Could you check a few things on this drawing? It's one solid part, dimensions in mm from its lowest x, y, z. A direction names the side the tool comes from. Give positions to 0.01 mm unless a question says otherwise; leave off trailing zeros. Order: outer loops, then holes, each group sorted by start corner. A loop starts at its lowest first (then second) coordinate and runs counter-clockwise, first axis right, second up.
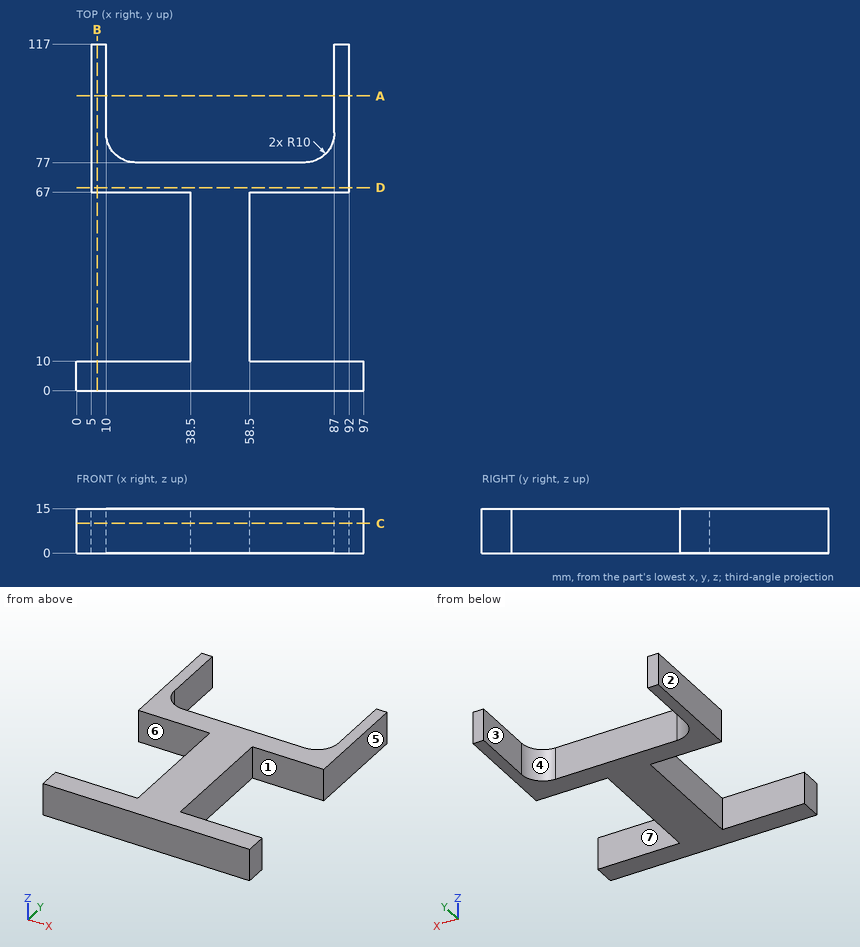
Item 1: Imagine slicing it at A-A on y = 99.5. List the corners of the cut face in (x, z) for me.
Findings:
outline: (5, 0) - (10, 0) - (10, 15) - (5, 15) - close; (87, 0) - (92, 0) - (92, 15) - (87, 15) - close
Item 2: For the marked faces 5, 6 and 7, which set-ups out of +Z, -Z, +X, -X, +Y, -Y let a thin tool reach every point of the face, with its end or its side?
Findings:
face 5: +Z, -Z, +X, +Y
face 6: +Z, -Z, -X
face 7: +Z, -Z, +X
Item 3: Imagine slicing it at D-D on y = 68.5. List the corners of the cut face in (x, z) for me.
Findings:
outline: (5, 0) - (92, 0) - (92, 15) - (5, 15) - close
Item 4: We'd pull the mould along X, two halves only. Please class the marked faces 1, 2, 3 and 4: +X half, -X half, draft (parallel to the pull), parting line (faces both ways), or undercut.
Findings:
face 1: draft
face 2: -X half
face 3: undercut
face 4: undercut
Item 5: Imagine slicing it at B-B on x = 7. List the corners of the cut face in (y, z) for me.
Findings:
outline: (0, 0) - (10, 0) - (10, 15) - (0, 15) - close; (67, 0) - (117, 0) - (117, 15) - (67, 15) - close
Item 6: Imagine slicing it at C-C on z = 10. List the corners of the cut face in (x, y) for me.
Findings:
outline: (0, 0) - (97, 0) - (97, 10) - (58.5, 10) - (58.5, 67) - (92, 67) - (92, 117) - (87, 117) - (87, 87) arc R10 cw to (77, 77) - (20, 77) arc R10 cw to (10, 87) - (10, 117) - (5, 117) - (5, 67) - (38.5, 67) - (38.5, 10) - (0, 10) - close
Item 7: For pin 1 (4.5 mm diameter, centred on y = 106, z = 8, fed in from +X); pin 2 (7.5 mm diameter, centred on x = 18.5, z = 5, fed in from +Y); pin 3 (4.5 mm diameter, centred on x = 83, z = 9.5, fed in from -Y); pin 4 (7.5 mm diameter, centred on x = 79, z = 7.5, fed in from +Y), each with a flat end and sliding along its axis, tell me the tip position at first contact or that it passes through.
Findings:
pin 1: stops at x = 92
pin 2: stops at y = 78.49
pin 3: stops at y = 0
pin 4: stops at y = 78.82
Item 8: Please list where these lines run through material, in increasing order: line 1 along X through (y, z) = (110, 13.5); line 2 along Y through (x, z) = (62, 12); line 3 along Y through (x, z) = (88, 8.5).
Findings:
line 1: x = 5 to 10, 87 to 92
line 2: y = 0 to 10, 67 to 77
line 3: y = 0 to 10, 67 to 117
